```python
from build123d import *

# Parameters (mm, degrees)
F1_DEPTH  = 1.524
F3_DEPTH  = 5.588
F4_R      = 1.4605
F5_DEPTH  = 1.143
F7_SIZE   = 0.508
F9_DEPTH  = 0.3175
F12_W     = 1.2032650411
F12_H     = 6.585133262
F12_W_2   = 0.508
F12_H_2   = 0.635
F13_DEPTH = 1.524
F14_R     = 1.524
F15_DEPTH = 25.4


# Not quite as in the source:
# - a fillet or chamfer that OpenCascade refuses, or shapes differently, is made with other operations: its cross-section is extruded or revolved along the edge and cut away or added


with BuildPart() as f1:
    # F0 (on Top) → F1 (new body)
    with BuildSketch(Plane.XY):
        Polygon((-17.78, -5.08), (13.97, -5.08), (16.4832153797, -2.5667846203), (7.62, -2.5667846203), (7.62, 2.5667846203), (16.4832153797, 2.5667846203), (13.97, 5.08), (-17.78, 5.08), align=None)
        Polygon((7.62, -2.5667846203), (16.4832153797, -2.5667846203), (17.78, -1.27), (17.78, 1.27), (16.4832153797, 2.5667846203), (7.62, 2.5667846203), align=None)
    extrude(amount=-F1_DEPTH)

    # F2 (on face) → F3 (join)
    with BuildSketch(Plane.XY):
        Polygon((16.4832153797, -2.5667846203), (17.78, -1.27), (17.78, 1.27), (16.4832153797, 2.5667846203), (7.62, 2.5667846203), (7.62, -2.5667846203), align=None)
    extrude(amount=F3_DEPTH)

    # F4 (on face) → F5 (join)
    with BuildSketch(Plane.XY.offset(5.588)):
        with Locations((10.829353705, 0)):
            Circle(F4_R)
        with Locations((14.7973923013, 0)):
            Circle(F4_R)
    extrude(amount=F5_DEPTH)

    # F6: fillet of radius 1.27 on 2 edges, made by hand

    # F6_s1 → F6_t2 (revolve, cut)
    with BuildSketch(Plane.XZ):
        with BuildLine():
            ThreePointArc((12.289853705, 5.588), (11.8781615594, 6.4028572079), (11.0262196599, 6.731))
            Line((11.0262196599, 6.731), (12.289853705, 6.731))
            Line((12.289853705, 6.731), (12.289853705, 5.588))
        make_face()
    revolve(axis=Axis((10.829353705, 0, 6.731), (0, 0, 1)), mode=Mode.SUBTRACT)

    # F6_s3 → F6_t4 (revolve, cut)
    with BuildSketch(Plane.XZ):
        with BuildLine():
            ThreePointArc((16.2578923013, 5.588), (15.8462001556, 6.4028572079), (14.9942582561, 6.731))
            Line((14.9942582561, 6.731), (16.2578923013, 6.731))
            Line((16.2578923013, 6.731), (16.2578923013, 5.588))
        make_face()
    revolve(axis=Axis((14.7973923013, 0, 6.731), (0, 0, 1)), mode=Mode.SUBTRACT)

    # F7
    f7_edges = [f1.edges().sort_by_distance(p)[0] for p in [
        (12.051608, -2.566785, 5.588),
        (12.051608, 2.566785, 5.588),
        (7.62, 0, 5.588),
        (17.78, 0, 5.588),
        (17.131608, -1.918392, 5.588),
        (17.131608, 1.918392, 5.588),
    ]]
    chamfer(f7_edges, length=F7_SIZE)

    # F11: F10_1 across plane


with BuildPart() as f9:
    # F8 (on Front) → F9 (new body, symmetric)
    with BuildSketch(Plane.XZ):
        with BuildLine():
            Line((-22.86, -5.334), (-22.86, -5.842))
            Line((-22.86, -5.842), (-15.9157037269, -5.842))
            ThreePointArc((-15.9157037269, -5.842), (-15.5230394847, -5.6793531454), (-15.3603926301, -5.2866889032))
            Line((-15.3603926301, -5.2866889032), (-15.3603926301, -1.1672781548))
            Line((-15.3603926301, -1.1672781548), (-15.8683926301, -1.1672781548))
            Line((-15.8683926301, -1.1672781548), (-15.8683926301, -5.334))
            Line((-15.8683926301, -5.334), (-22.86, -5.334))
        make_face()
    extrude(amount=F9_DEPTH, both=True)


with BuildPart() as f10_1:
    # F10: copy of F9
    add(f9.part.moved(Location((0, -2.54, 0))))


with BuildPart() as f1_1:
    add(f1.part)
    add(f10_1.part.mirror(Plane.XZ))


    add(f9.part)  # F13 merges F9

    add(f10_1.part)  # F13 merges F10_1
    # F12 (on face) → F13 (join)
    with BuildSketch(Plane(origin=(0, 0, -1.524), x_dir=(1, 0, 0), z_dir=(0, 0, -1))):
        with Locations((-15.6205464154, 0)):
            Rectangle(F12_W, F12_H)
        with Locations((-15.6143926301, -2.54)):
            Rectangle(F12_W_2, F12_H_2, mode=Mode.SUBTRACT)
    extrude(amount=F13_DEPTH)

    # F14 (on face) → F15 (cut)
    with BuildSketch(Plane(origin=(0, 0, -1.524), x_dir=(1, 0, 0), z_dir=(0, 0, -1))):
        with Locations((-0.254, 0)):
            Circle(F14_R)
    extrude(amount=-F15_DEPTH, mode=Mode.SUBTRACT)


solid = f1_1.part
```
For this review, take the finished solid that the model builds, in its own axes (mm). A direction names the side the tool comes from. Round coordinates to 2 decimals unless told otherwise and drop trailing zeros. Write each loop counter-clockwise with the first axis right and the second up, starting at its lowest first coordinate (ties: lowest second). Pieces come first, ordered by that corner, then holes. Notation, with made-up numbers: (55, 74.25) -> (66, 74.25) arc R29 ccw to (66, 111.25) -> close; hole circle Ø1 at (79, 41). An arc over 180 degrees is marked (long way). Use one line per item in the form item = value.
1) Take a section at B-B, the plane z = -2. Write out the cut boundary in (x, y).
Found:
outline = (-16.22, -3.29) -> (-15.02, -3.29) -> (-15.02, 3.29) -> (-16.22, 3.29) -> close
2) Take a section at D-D, the plane x = -9. Write out the cut boundary in (y, z), and give its area (3 significant figures).
Found:
outline = (-5.08, -1.52) -> (5.08, -1.52) -> (5.08, 0) -> (-5.08, 0) -> close
area = 15.5 mm2
3) Take a section at C-C, the plane x = -1. Write out the cut boundary in (y, z).
Found:
outline = (-5.08, -1.52) -> (-1.33, -1.52) -> (-1.33, 0) -> (-5.08, 0) -> close; (1.33, -1.52) -> (5.08, -1.52) -> (5.08, 0) -> (1.33, 0) -> close
4) Mouldability with a two-part tool opening along Y and no side actions: class faces 4 (the flat face through (12, -2.567, 3)), 5 (the cylindrical face through (-0.45, -1.51, -0.77)), 6 (the flat face through (-15.019, 0, -2)) as +Y half, -Y half, draft (parallel to the pull), parting line (faces both ways), or undercut.
Found:
face_4 = -Y half
face_5 = undercut
face_6 = draft
5) Take a section at A-A, the plane x = -18.5. Write out the cut boundary in (y, z), and give its area (3 significant figures).
Found:
outline = (-2.86, -5.84) -> (-2.22, -5.84) -> (-2.22, -5.33) -> (-2.86, -5.33) -> close; (-0.32, -5.84) -> (0.32, -5.84) -> (0.32, -5.33) -> (-0.32, -5.33) -> close; (2.22, -5.84) -> (2.86, -5.84) -> (2.86, -5.33) -> (2.22, -5.33) -> close
area = 0.968 mm2
6) To check wall thickness, follow L1, parallel to X at y = 0, z = -0.7; L2, parallel to Z at x = -12.5, y = 2.75; L3, parallel to X at y = 2.5, z = -2.5. State the ranges of each line that lie inside material, in increasing order. Write a range as from..to.
Found:
L1 = -17.78..-1.78, 1.27..17.78
L2 = -1.52..0
L3 = -16.22..-15.02
7) Clearance check with flat-ended pins moving along their axes: pin 1 (6 mm diameter, centred on y = 1, z = -2, fed in from -X); pin 2 (0.6 mm diameter, centred on x = -15.5, z = -2, fed in from -Y); pin 3 (6 mm diameter, centred on x = -10, z = 5.5, fed in from +Y); pin 4 (0.5 mm diameter, centred on y = 0, z = -4, fed in from -X). State where each tip first meets the part, or that it passes through.
Found:
pin_1 = -17.78
pin_2 = -3.29
pin_3 = through
pin_4 = -15.87
8) Tool access review of faces 1 (the flat face through (-16.222, 0, -2)), 2 (the flat face through (13, 0, 5.588)), 3 (the flat face through (-18.3, -2.858, -5.5)): name each direction out of +Z, -Z, +X, -X, +Y, -Y from which nothing blocks a thin tool from reaching the whole face with its end or side.
Found:
face_1 = -X, +Y, -Y
face_2 = +Z
face_3 = -Z, +X, -X, -Y
